The listing builds one solid part. Answer for the finished solid, in the listing's coordinates (mm). Give positions to 0.01 mm unless a question says otherwise; leave off trailing zeros. Write each loop counter-clockwise with the first axis right and the second up, starting at its lowest first coordinate (ties: lowest second). Pieces come first, ordered by that corner, then holes. Notation, with made-up numbers: M -2.75,52.5 L 6.25,52.5 A25 ccw 6.25,72.5 Z; hole C -5.75,10 d11. An arc over 180 degrees is marked long. Return JSON: item names as keys, results as strings.
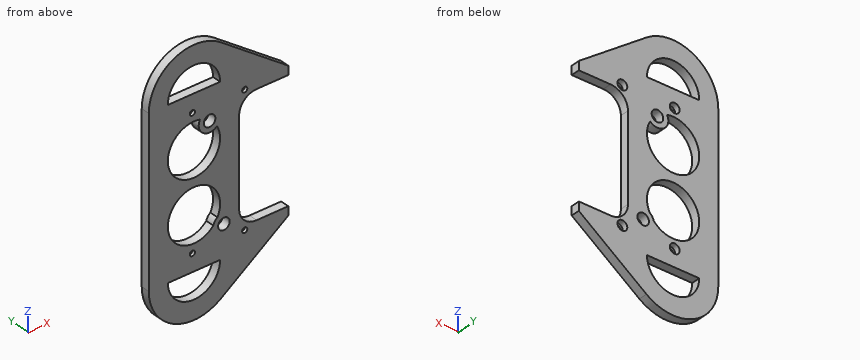
from build123d import *

# Parameters (mm, degrees)
BOSS_EXTRUDE1_DEPTH                            = 6.35
FILLET1_R                                      = 12.7
TAP_DRILL_FOR_3_8_24_TAP1_D                    = 8.4328
CBORE_FOR_6_SOCKET_HEAD_CAP_SCREW1_D           = 3.7973
CBORE_FOR_6_SOCKET_HEAD_CAP_SCREW1_CBORE_D     = 7.14502
CBORE_FOR_6_SOCKET_HEAD_CAP_SCREW1_CBORE_DEPTH = 4.0132


with BuildPart() as part:
    # Sketch1 → Boss-Extrude1 (new body)
    with BuildSketch(Plane(origin=(0, 53.278467802, 0), x_dir=(1, 0, 0), z_dir=(0, 1, 0))):
        with BuildLine():
            ThreePointArc((-14.919754069, 137.471595351), (-49.255675468, 140.270872374), (-67.283137827, 110.914407139))
            Line((-67.283137827, 110.914407139), (-67.283137827, -9.525))
            ThreePointArc((-67.283137827, -9.525), (-49.255676138, -38.881464895), (-14.919755281, -36.0821891))
            Line((-14.919755281, -36.0821891), (34.354322218, 0))
            Line((34.354322218, 0), (34.354322218, 6.35))
            Line((34.354322218, 6.35), (-1.450719122, 6.35))
            Line((-1.450719122, 6.35), (-1.450719122, 95.039403682))
            Line((-1.450719122, 95.039403682), (34.354322218, 95.039403682))
            Line((34.354322218, 95.039403682), (34.354322218, 101.389403682))
            Line((34.354322218, 101.389403682), (-14.919754069, 137.471595351))
        make_face()
        with BuildLine():
            Line((-53.416928475, -9.525), (-34.366928475, -9.525))
            Line((-34.366928475, -9.525), (-15.316928475, -9.525))
            ThreePointArc((-15.316928475, -9.525), (-34.366928475, -28.575), (-53.416928475, -9.525))
        make_face(mode=Mode.SUBTRACT)
        with BuildLine():
            ThreePointArc((-29.961916932, 9.935994461), (-46.001401892, 43.554183286), (-17.560004644, 19.501436661))
            ThreePointArc((-17.560004644, 19.501436661), (-27.817615961, 19.978303209), (-29.961916932, 9.935994461))
        make_face(mode=Mode.SUBTRACT)
        with BuildLine():
            ThreePointArc((-17.256926776, 81.295283661), (-50.136649325, 62.232402493), (-20.247770765, 85.708444148))
            ThreePointArc((-20.247770765, 85.708444148), (-19.133936144, 83.24325824), (-17.256926776, 81.295283661))
        make_face(mode=Mode.SUBTRACT)
        with BuildLine():
            Line((-34.366928475, 110.914407139), (-53.416928475, 110.914407139))
            ThreePointArc((-53.416928475, 110.914407139), (-34.366928475, 129.964407139), (-15.316928475, 110.914407139))
            Line((-15.316928475, 110.914407139), (-34.366928475, 110.914407139))
        make_face(mode=Mode.SUBTRACT)
    extrude(amount=BOSS_EXTRUDE1_DEPTH)

    # Fillet1
    fillet1_edges = [part.edges().sort_by_distance(p)[0] for p in [
        (-1.450719122, 56.453467802, -6.35),
        (-1.450719122, 56.453467802, -95.039403682),
    ]]
    fillet(fillet1_edges, radius=FILLET1_R)

    # Tap Drill for 3/8-24 Tap1 (through all)
    with Locations(Plane(origin=(0, 59.628467802, 0), x_dir=(1, 0, 0), z_dir=(0, 1, 0))):
        with Locations((-22.969918704, 13.693103328), (-12.563219122, 87.696300355)):
            Hole(TAP_DRILL_FOR_3_8_24_TAP1_D / 2)

    # CBORE for #6 Socket Head Cap Screw1 (through all)
    with Locations(Plane(origin=(0, 59.628467802, 0), x_dir=(1, 0, 0), z_dir=(0, 1, 0))):
        with Locations((2.604322218, 3.175), (-35.533137827, 3.175), (-35.533137827, 98.214403682), (2.604322218, 98.214403682)):
            CounterBoreHole(CBORE_FOR_6_SOCKET_HEAD_CAP_SCREW1_D / 2, CBORE_FOR_6_SOCKET_HEAD_CAP_SCREW1_CBORE_D / 2, CBORE_FOR_6_SOCKET_HEAD_CAP_SCREW1_CBORE_DEPTH)


solid = part.part
Item 1: Find the intervals of material crossed by line 1 (Z direction, x = -17.5, y = 56.25) (3 decimals); line 2 (X direction, y = 54.75, z = -28); line 3 (Z direction, x = -20.5, y = 54.5) (3 decimals), in increasing order.
Geometry results:
{"line 1": "z = -139.181 to -119.769, -110.914 to -81.481, -64.065 to -37.325, -19.615 to 9.525, 18.38 to 37.791", "line 2": "x = -67.28 to -53.41, -15.32 to -1.45", "line 3": "z = -140.767 to -123.976, -110.914 to -85.982, -59.858 to -41.532, -21.237 to -17.11, -10.276 to 9.525, 22.587 to 39.378"}
Item 2: A cutting plane is placed at B-B, the plane y = 54.25. Count the separate pieces of the cut face and the enclosed holes in it, plus the area to 3 significant figures.
Geometry results:
{"separate pieces": "1", "enclosed holes": "10", "area": "9,400 mm2"}
Item 3: Given pin 1 Ø1.9 at (x, y) = (22, 55) entering from -Z; pin 2 Ø2 at (x, y) = (-37.5, 55) entering from -Z; pin 3 Ø3 at (x, y) = (-44, 58) entering from +Z, each flat-ended and moving along its own axis, determine where each tip first touches the part or whether it passes through.
Geometry results:
{"pin 1": "stops at z = -111.13", "pin 2": "stops at z = -143.76", "pin 3": "stops at z = 41.42"}
Item 4: A cutting plane is placed at C-C, the plane x = -50. Write down the section's boundary in (y, z) (1 decimal).
Geometry results:
{"outline": "M 53.3,-139.9 L 59.6,-139.9 L 59.6,-121.8 L 53.3,-121.8 Z; M 53.3,-110.9 L 59.6,-110.9 L 59.6,-83.8 L 53.3,-83.8 Z; M 53.3,-62 L 59.6,-62 L 59.6,-39.4 L 53.3,-39.4 Z; M 53.3,-17.6 L 59.6,-17.6 L 59.6,9.5 L 53.3,9.5 Z; M 53.3,20.4 L 59.6,20.4 L 59.6,38.5 L 53.3,38.5 Z"}
Item 5: A cutting plane is placed at A-A, the plane z = 24. Write down the section's boundary in (x, y), plus the area to 3 significant figures.
Geometry results:
{"outline": "M -63.93,53.28 L -46.75,53.28 L -46.75,59.63 L -63.93,59.63 Z; M -21.98,53.28 L 1.58,53.28 L 1.58,59.63 L -21.98,59.63 Z", "area": "259 mm2"}
Item 6: A cutting plane is placed at D-D, the plane x = -13. Write down the section's boundary in (y, z).
Geometry results:
{"outline": "M 53.28,-136.07 L 59.63,-136.07 L 59.63,-91.89 L 53.28,-91.89 Z; M 53.28,-83.5 L 59.63,-83.5 L 59.63,34.68 L 53.28,34.68 Z"}
